Source: three-view drawing plus pictorial views. Frame: mm from the lowest corner of the part. Round coordinates to 2 decimals unless told otherwise and drop trailing zeros. Loops run counter-clockwise (first coordinate to the right, second up) from the corner with the lowest first, then second, coordinate; pieces in that order, holes last. Notation, with made-up numbers: M 84.25,-40 L 108.25,-40 A33 cw 108.25,-1 Z; hole C 42.25,83 d8. An arc over 180 degrees is marked long. Write each question's results on one line, items separated by ' | '.
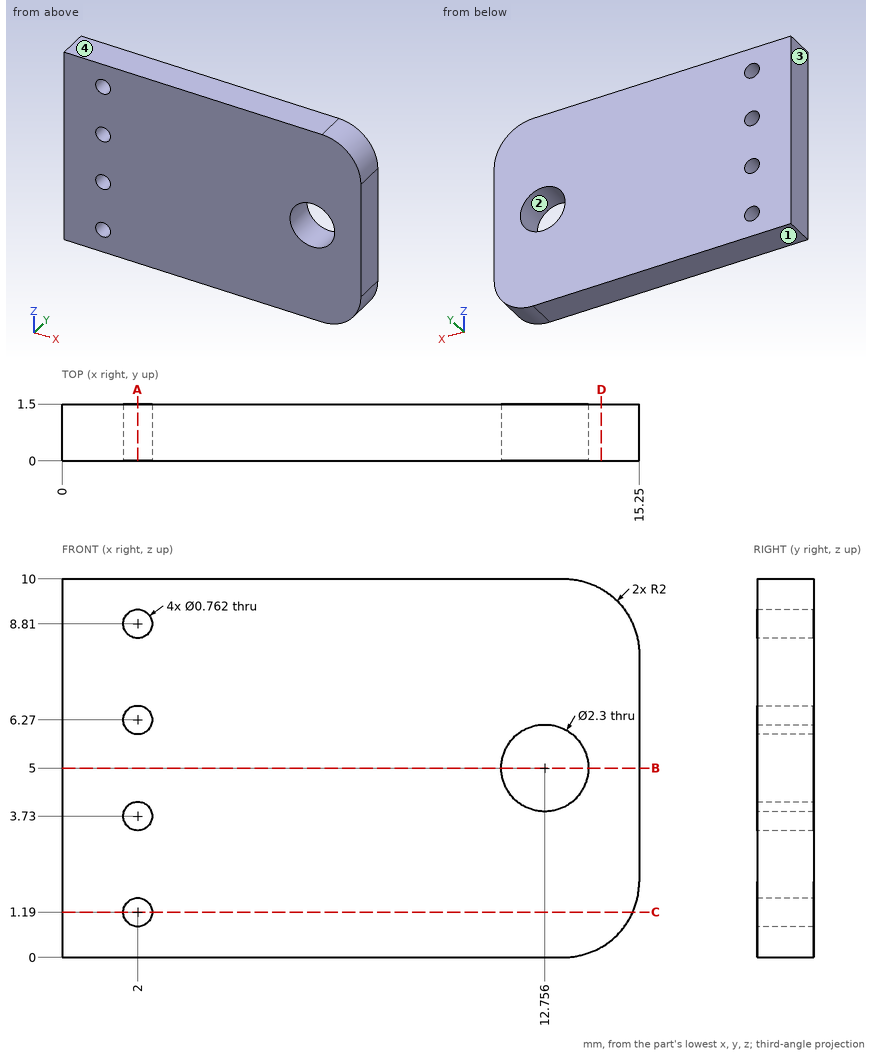
1. Section C-C (z = 1.19). Output: boundary loops of the cut face in (x, y).
Answer key:
outline: M 0,0 L 1.62,0 L 1.62,1.5 L 0,1.5 Z; M 2.38,0 L 15.08,0 L 15.08,1.5 L 2.38,1.5 Z
2. Ray query, probe 1 along X at (y, z) = (1.1, 6.27); probe 2 along Z at (x, y) = (1.75, 0.6); probe 3 along Z at (x, y) = (13.75, 0.8) (1 decimal). Return the intervals inside material, ascending.
Answer key:
probe 1: x = 0 to 1.62, 2.38 to 15.25 | probe 2: z = 0 to 0.9, 1.48 to 3.44, 4.02 to 5.98, 6.56 to 8.52, 9.1 to 10 | probe 3: z = 0.1 to 4.4, 5.6 to 9.9
3. Section B-B (z = 5). Output: boundary loops of the cut face in (x, y), then the cut area to 3 significant figures.
Answer key:
outline: M 0,0 L 11.61,0 L 11.61,1.5 L 0,1.5 Z; M 13.91,0 L 15.25,0 L 15.25,1.5 L 13.91,1.5 Z | area: 19.4 mm²
4. Section A-A (x = 2). Output: boundary loops of the cut face in (y, z).
Answer key:
outline: M 0,0 L 1.5,0 L 1.5,0.81 L 0,0.81 Z; M 0,1.57 L 1.5,1.57 L 1.5,3.35 L 0,3.35 Z; M 0,4.11 L 1.5,4.11 L 1.5,5.89 L 0,5.89 Z; M 0,6.65 L 1.5,6.65 L 1.5,8.43 L 0,8.43 Z; M 0,9.19 L 1.5,9.19 L 1.5,10 L 0,10 Z
5. Section D-D (x = 14.25). Output: boundary loops of the cut face in (y, z).
Answer key:
outline: M 0,0.27 L 1.5,0.27 L 1.5,9.73 L 0,9.73 Z
6. Draft query along Z for the marked faces 1, 2, 3 and 4. Return one class per face: pulls with the +Z half, pulls with the -Z half, needs draft (parallel to the pull), parting line crosses it, or undercut.
Answer key:
face 1: pulls with the -Z half | face 2: undercut | face 3: needs draft | face 4: pulls with the +Z half
